Design review of the part built by this model. Coordinates are the model's own, in mm. Coordinates: 2 decimals unless noted, no trailing zeros. Loops run counter-clockwise (first coordinate to the right, second up) from the corner with the lowest first, then second, coordinate; pieces in that order, holes last. Notation, with made-up numbers: (34, -0.75) -> (46, -0.75) arc R26 ccw to (46, 32.25) -> close; hole circle Ø7 at (-11, 58.5). An arc over 180 degrees is marked (long way). One line per item, written item: value. Start each with the question number.
1. Add section B-B on y = 204. Write out the cut boundary in (x, z).
2. For probe 1 along X at (y, z) = (393, 4.5); probe 2 along Y at (x, z) = (164.5, 3.75), list the stretches that pass through material, from the lowest coordinate up.
3. Add section A-A on x = 179. Write out the cut boundary in (y, z), plus the area to 3 significant figures.
4. Insertion check: pin 1 (3 mm diameter, centred on x = 3.5, z = 3.5, fed in from +Y); pin 2 (3 mm diameter, centred on x = 263.5, z = 2.5, fed in from -Y); pin 3 (1.9 mm diameter, centred on x = 171.5, z = 3.5, fed in from -Y); pin 4 (2 mm diameter, centred on x = 28.5, z = 0.5, fed in from -Y). Each pin has a flat end and moves straight along its axis. Give the tip position at first contact, or say it passes through.
```python
from build123d import *

# Parameters (mm, degrees)
BOSS_EXTRUDE1_DEPTH = 6.35


with BuildPart() as part:
    # Sketch1 → Boss-Extrude1 (new body)
    with BuildSketch(Plane.XY):
        Polygon((6.35, 521.67), (6.35, 470.87), (0, 470.87), (0, 420.07), (6.35, 420.07), (6.35, 369.27), (0, 369.27), (0, 318.47), (6.35, 318.47), (6.35, 267.67), (0, 267.67), (0, 216.87), (6.35, 216.87), (6.35, 166.07), (0, 166.07), (0, 115.27), (6.35, 115.27), (6.35, 64.47), (0, 64.47), (0, 13.67), (6.35, 13.67), (6.35, 0), (50.8, 0), (50.8, 6.35), (101.6, 6.35), (101.6, 0), (152.4, 0), (152.4, 6.35), (203.2, 6.35), (203.2, 0), (254, 0), (260.35, 0), (260.35, 6.35), (260.35, 13.67), (266.7, 13.67), (266.7, 64.47), (260.35, 64.47), (260.35, 115.27), (266.7, 115.27), (266.7, 166.07), (260.35, 166.07), (260.35, 216.87), (266.7, 216.87), (266.7, 267.67), (260.35, 267.67), (260.35, 318.47), (266.7, 318.47), (266.7, 369.27), (260.35, 369.27), (260.35, 420.07), (266.7, 420.07), (266.7, 470.87), (260.35, 470.87), (260.35, 521.67), (254, 521.67), (203.2, 521.67), (203.2, 515.32), (152.4, 515.32), (152.4, 521.67), (101.6, 521.67), (101.6, 515.32), (50.8, 515.32), (50.8, 521.67), align=None)
    extrude(amount=BOSS_EXTRUDE1_DEPTH)


solid = part.part
```
Worked answers:
1. outline: (6.35, 0) -> (260.35, 0) -> (260.35, 6.35) -> (6.35, 6.35) -> close
2. probe 1: x = 6.35 to 260.35
2. probe 2: y = 6.35 to 515.32
3. outline: (6.35, 0) -> (515.32, 0) -> (515.32, 6.35) -> (6.35, 6.35) -> close
3. area: 3,230 mm²
4. pin 1: stops at y = 470.87
4. pin 2: stops at y = 13.67
4. pin 3: stops at y = 6.35
4. pin 4: stops at y = 0
